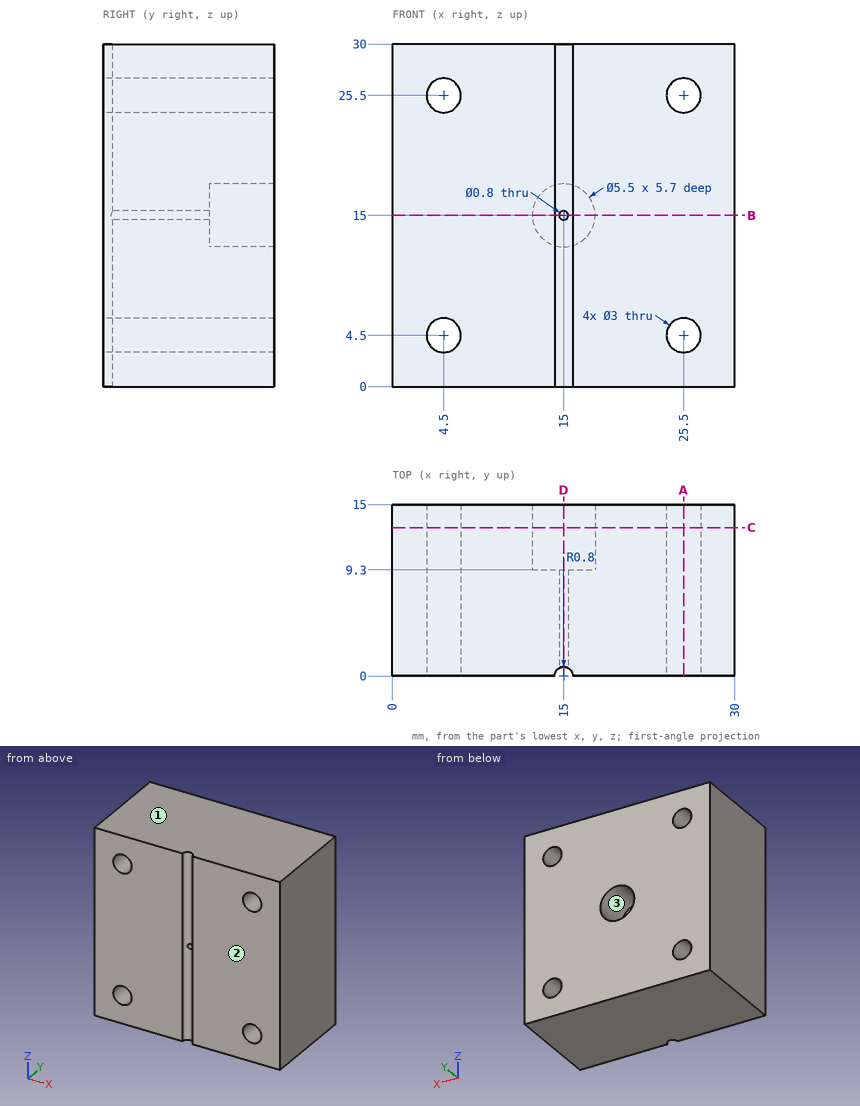
Answer from the drawing. Dimensions are ordinates in mm from the lowest x, y and z of the part. Round coordinates to 2 decimals unless told otherwise and drop trailing zeros. Order: outer loops, then holes, each group sorted by start corner. A loop starts at its lowest first (then second) coordinate and runs counter-clockwise, first axis right, second up. Notation, with made-up numbers: (41.25, 15.25) - (82.25, 15.25) arc R7 ccw to (82.25, 25.25) - close; hole circle Ø4 at (22, 29.5). An arc over 180 degrees is marked (long way). Put each result on its own line as item: value. Start each with the question number.
(1) Straight lines are drawn through the part: probe 1 along Z at (x, y) = (4.5, 10.75); probe 2 along Z at (x, y) = (15, 10.8). For each, find the intervals that lie inside material, in ascending order. Write a range as from..to.
(2) Determine the mould class of the marked faces 1, 2 and 3 for opening direction Z: released by +Z, released by -Z, zero draft, split by the parting line, or undercut.
(3) Find section D-D (x = 15). Give the vertices of the cut face in (y, z).
(4) Given P1, Ø2.5, axis at x = 4.5, z = 25.5, coming from the -Y side, flat-ended and moving along its own axis, determine where the tip first touches the part or whether it passes through.
(5) Find section C-C (y = 13). Give the vertices of the cut face in (x, z).
(6) Find section B-B (z = 15). Give the vertices of the cut face in (x, y), plus the area to 3 significant figures.
(7) Find section A-A (x = 25.5). Give the vertices of the cut face in (y, z).
Reply:
1. probe 1: 0..3, 6..24, 27..30
1. probe 2: 0..12.25, 17.75..30
2. face 1: released by +Z
2. face 2: zero draft
2. face 3: undercut
3. outline: (0.8, 0) - (15, 0) - (15, 12.25) - (9.3, 12.25) - (9.3, 14.6) - (0.8, 14.6) - close; (0.8, 15.4) - (9.3, 15.4) - (9.3, 17.75) - (15, 17.75) - (15, 30) - (0.8, 30) - close
4. P1: through
5. outline: (0, 0) - (30, 0) - (30, 30) - (0, 30) - close; hole circle Ø3 at (4.5, 4.5); hole circle Ø3 at (4.5, 25.5); hole circle Ø5.5 at (15, 15); hole circle Ø3 at (25.5, 4.5); hole circle Ø3 at (25.5, 25.5)
6. outline: (0, 0) - (14.2, 0) arc R0.8 cw to (14.6, 0.69) - (14.6, 9.3) - (12.25, 9.3) - (12.25, 15) - (0, 15) - close; (15.4, 0.69) arc R0.8 cw to (15.8, 0) - (30, 0) - (30, 15) - (17.75, 15) - (17.75, 9.3) - (15.4, 9.3) - close
6. area: 411 mm^2
7. outline: (0, 0) - (15, 0) - (15, 3) - (0, 3) - close; (0, 6) - (15, 6) - (15, 24) - (0, 24) - close; (0, 27) - (15, 27) - (15, 30) - (0, 30) - close
